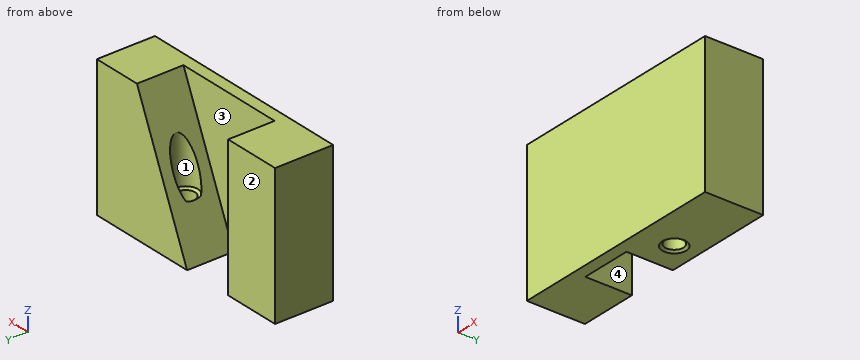
from build123d import *

# Parameters (mm, degrees)
SKETCH_3_W            = 19
SKETCH_3_H            = 12
EXTRUDE_1_DEPTH       = 5
HOLE_WIZARD_M23_D     = 2.1
HOLE_WIZARD_M23_DEPTH = 8
HOLE_WIZARD_M23_TIP   = 0.63090365
CUT_EXTRUDE_1_DEPTH   = 4


with BuildPart() as part:
    # Эскиз3 → Бобышка-Вытянуть1 (new body)
    with BuildSketch(Plane(origin=(0, 0, 0), x_dir=(1, 0, 0), z_dir=(0, 1, 0))):
        with Locations((9.5, 6)):
            Rectangle(SKETCH_3_W, SKETCH_3_H)
    extrude(amount=EXTRUDE_1_DEPTH)

    # Эскиз8 → Отверстие обработанное метчиком M2x0.42 (revolve, cut)
    with BuildSketch(Plane(origin=(12, 3, -12), x_dir=(0, 1, 0), z_dir=(1, 0, 0))):
        Polygon((0, 0), (0, 12), (1.025, 12), (0.8, 11.842453304), (0.8, 0.157546696), (1.025, 0), align=None)
    revolve(axis=Axis((12, 3, -18.35), (0, 0, 1)), mode=Mode.SUBTRACT)

    # Отверстие с зазором M23
    with Locations(Plane.XY):
        with Locations((12, 3)):
            Hole(HOLE_WIZARD_M23_D / 2, depth=HOLE_WIZARD_M23_DEPTH)
            with Locations((0, 0, -(HOLE_WIZARD_M23_DEPTH + HOLE_WIZARD_M23_TIP / 2))):  # 118° drill point
                Cone(0, HOLE_WIZARD_M23_D / 2, HOLE_WIZARD_M23_TIP, mode=Mode.SUBTRACT)

    # Эскиз4 → Вырез-Вытянуть1 (cut)
    with BuildSketch(Plane(origin=(0, 5, 0), x_dir=(1, 0, 0), z_dir=(0, 1, 0))):
        Polygon((5, 12), (5, 0), (14.721289338, 0), (9.378545114, 12), align=None)
    extrude(amount=-CUT_EXTRUDE_1_DEPTH, mode=Mode.SUBTRACT)


solid = part.part
Design review of the part built by this model. Coordinates are the model's own, in mm. Face numbers are marked on the shaded views. A direction names the side the tool comes from. Coordinates: 2 decimals unless noted, no trailing zeros. Loops run counter-clockwise (first coordinate to the right, second up) from the corner with the lowest first, then second, coordinate; pieces in that order, holes last.
Item 1: Add section B-B (x = 12). Write out the cut boundary in (y, z) (3 decimals).
Completed:
outline: (0, -12) - (1.975, -12) - (2.2, -11.842) - (2.2, -8.15) - (1.95, -8) - (1.95, -6.112) - (1, -6.112) - (1, 0) - (0, 0) - close; (3.8, -11.842) - (4.025, -12) - (5, -12) - (5, -6.112) - (4.05, -6.112) - (4.05, -8) - (3.8, -8.15) - close
Item 2: Add section A-A (y = 3). Write out the cut boundary in (x, z) (3 decimals).
Completed:
outline: (0, -12) - (5, -12) - (5, 0) - (0, 0) - close; (9.379, -12) - (10.975, -12) - (11.2, -11.842) - (11.2, -8.15) - (11.115, -8.099) - close; (12.8, -11.842) - (13.025, -12) - (19, -12) - (19, 0) - (14.721, 0) - (13.05, -3.754) - (13.05, -8) - (12.8, -8.15) - close
Item 3: For the marked faces 1, 2, 3 and 4, list the 3-axis set-ups (+Z, -Z, +X, -X, +Y, -Y) from which the entire face can be reached by the end or side of a thin tool; tool diameter is ignored.
Completed:
face 1: +Z
face 2: +Z, -Z, +X, -X, +Y
face 3: +Z, +Y
face 4: +Z, -Z, +Y
Item 4: Add section C-C (z = -1.25). Write out the cut boundary in (x, y), and give its area (3 significant figures).
Completed:
outline: (0, 0) - (19, 0) - (19, 5) - (14.16, 5) - (14.16, 1) - (5, 1) - (5, 5) - (0, 5) - close
area: 58.3 mm2
Item 5: Clearance check with flat-ended pins moving along their axes: pin 1 (4 mm diameter, centred on x = 5.5, z = -5.5, fed in from -Y); pin 2 (1 mm diameter, centred on x = 12, y = 3, fed in from -Z). State where each tip first meets the part, or that it passes through.
Completed:
pin 1: stops at y = 0
pin 2: passes through
Item 6: Wall thickness on L1, parallel to X at y = 3, z = -5; L2, parallel to Y at x = 12, z = -10.8; L3, parallel to Y at x = 12, z = -7: over which ranges is each line inside the solid? List them lowest first.
Completed:
L1: x = 0 to 5, 13.05 to 19
L2: y = 0 to 2.2, 3.8 to 5
L3: y = 0 to 1.95, 4.05 to 5
Item 7: Add section D-D (z = -8.5). Write out the cut boundary in (x, y), and give its area (3 significant figures).
Completed:
outline: (0, 0) - (19, 0) - (19, 5) - (10.94, 5) - (10.94, 1) - (5, 1) - (5, 5) - (0, 5) - close; hole circle Ø1.6 at (12, 3)
area: 69.2 mm2
